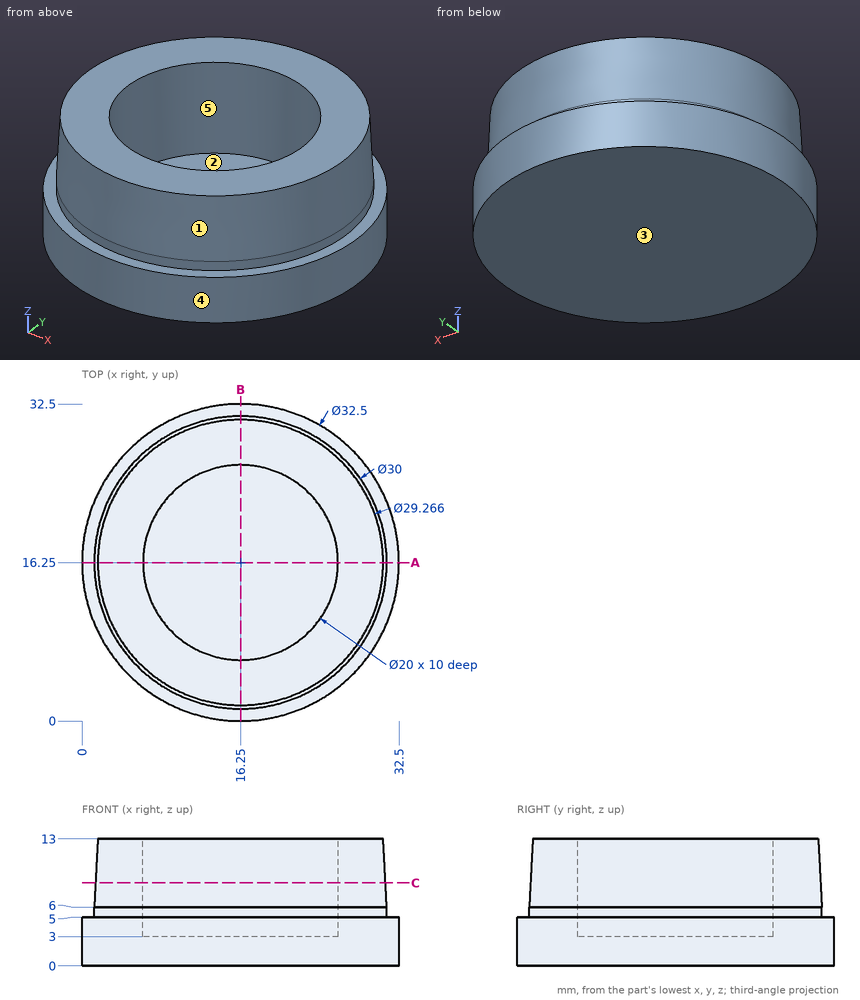
Input: dimensioned drawing with shaded views. Units: mm. Origin: part minimum x, y, z. A direction names the side the tool comes from. Give positions to 0.01 mm unless a question says otherwise; leave off trailing zeros. Write each loop counter-clockwise with the first axis right and the second up, starting at its lowest first coordinate (ties: lowest second). Pieces come first, ordered by that corner, then holes. Notation, with made-up numbers: (70, 5) -> (112, 5) arc R22 cw to (112, 21) -> close; hole circle Ø7 at (33, -28). An arc over 180 degrees is marked (long way). Answer as a JSON object with one key per item and string values.
1. Access query for the marked faces 4 and 5. Directions: +Z, -Z, +X, -X, +Y, -Y. A direction counts if a zero-diameter tool reaches every point of the face in a straight line with its end or side. Return the directions, or none.
Ans:
{"face 4": "+Z, -Z", "face 5": "+Z"}
2. Ray query, probe 1 along Z at (x, y) = (20, 17.5); probe 2 along X at (y, z) = (15.5, 9.5); probe 3 along Y at (x, z) = (19, 6.5) (1 decimal). Return the intervals inside material, ascending. Write a range as from..to.
Ans:
{"probe 1": "z = 0..3", "probe 2": "x = 1.45..6.28, 26.22..31.05", "probe 3": "y = 1.5..6.6, 25.9..31"}
3. Cut plane C-C on z = 8.5. Output: boundary loops of the cut face in (x, y).
Ans:
{"outline": "circle Ø29.74 at (16.25, 16.25); hole circle Ø20 at (16.25, 16.25)"}
4. Contact query for flat-ended pins moving along their axis: pin 1 (6 mm diameter, centred on y = 13, z = 4.5, fed in from +X); pin 2 (6 mm diameter, centred on x = 14, y = 16, fed in from +Z); pin 3 (3 mm diameter, centred on x = 10.5, z = 8, fed in from +Y). Output: stop coordinate, or through.
Ans:
{"pin 1": "stops at x = 32.5", "pin 2": "stops at z = 3", "pin 3": "stops at y = 30.53"}
5. Mould query, pull axis X, two halves, no side actions, for the marked faces 1, 2 and 3. Classes: pulls with the +X half, pulls with the -X half, needs draft (parallel to the pull), parting line crosses it, or undercut.
Ans:
{"face 1": "parting line crosses it", "face 2": "undercut", "face 3": "needs draft"}
6. Cut plane A-A on y = 16.25. Output: boundary loops of the cut face in (x, z), and give its area (3 significant figures).
Ans:
{"outline": "(0, 0) -> (32.5, 0) -> (32.5, 5) -> (31.25, 5) -> (31.25, 6) -> (30.88, 13) -> (26.25, 13) -> (26.25, 3) -> (6.25, 3) -> (6.25, 13) -> (1.62, 13) -> (1.25, 6) -> (1.25, 5) -> (0, 5) -> close", "area": "200 mm^2"}
